```python
from build123d import *

# Parameters (mm, degrees)
SKETCH1_W           = 60
SKETCH1_H           = 12
BOSS_EXTRUDE1_DEPTH = 18.5
SKETCH2_W           = 65
SKETCH2_H           = 6.6
CUT_EXTRUDE1_DEPTH  = 15
SKETCH3_R           = 1.6
CUT_EXTRUDE2_DEPTH  = 38.232378382
CUT_EXTRUDE3_DEPTH  = 37.451886097
FILLET1_R           = 0.7
FILLET3_R           = 0.7
FILLET4_R           = 3
SKETCH5_R           = 1.5
CUT_EXTRUDE4_DEPTH  = 35.073450224
FILLET5_R           = 0.5
SKETCH6_W           = 73.746826028
SKETCH6_H           = 28.597179554
CUT_EXTRUDE5_DEPTH  = 2
SKETCH8_R           = 1.5
BOSS_EXTRUDE2_DEPTH = 0.7


with BuildPart() as part:
    # Sketch1 → Boss-Extrude1 (new body)
    with BuildSketch(Plane.XY):
        Rectangle(SKETCH1_W, SKETCH1_H)
    extrude(amount=BOSS_EXTRUDE1_DEPTH)

    # Sketch2 → Cut-Extrude1 (cut)
    with BuildSketch(Plane.XY.offset(18.5)):
        Rectangle(SKETCH2_W, SKETCH2_H)
    extrude(amount=-CUT_EXTRUDE1_DEPTH, mode=Mode.SUBTRACT)

    # Sketch3 → Cut-Extrude2 (cut, through all)
    with BuildSketch(Plane(origin=(0, 6, 0), x_dir=(1, 0, 0), z_dir=(0, 1, 0))):
        with Locations(Location((25, -15.5, 0), (0, 0, 180))):
            Circle(SKETCH3_R)
        with Locations(Location((-25, -15.5, 0), (0, 0, 180))):
            Circle(SKETCH3_R)
    extrude(amount=-CUT_EXTRUDE2_DEPTH, mode=Mode.SUBTRACT)

    # Sketch4 → Cut-Extrude3 (cut, symmetric)
    with BuildSketch(Plane(origin=(0, -3.3, 0), x_dir=(1, 0, 0), z_dir=(0, 1, 0))):
        Polygon((-30, -3.5), (-28, -18.5), (-30, -18.5), align=None)
    cut_extrude3 = extrude(amount=CUT_EXTRUDE3_DEPTH, both=True, mode=Mode.SUBTRACT)

    # Mirror1: Cut-Extrude3 across plane
    add(cut_extrude3.mirror(Plane(origin=(0, 0, 0), x_dir=(0, 0, 1), z_dir=(1, 0, 0))), mode=Mode.SUBTRACT)

    # Fillet1
    fillet1_edges = [part.edges().sort_by_distance(p)[0] for p in [
        (0, 3.3, 3.5),
        (0, -3.3, 3.5),
    ]]
    fillet(fillet1_edges, radius=FILLET1_R)

    # Fillet3
    fillet3_edges = [part.edges().sort_by_distance(p)[0] for p in [
        (0, -3.3, 18.5),
        (0, -6, 18.5),
        (-28, 4.65, 18.5),
        (-28, -4.65, 18.5),
        (0, 3.3, 18.5),
        (0, 6, 18.5),
        (28, 4.65, 18.5),
        (28, -4.65, 18.5),
    ]]
    fillet(fillet3_edges, radius=FILLET3_R)

    # Fillet4
    # the kernel refuses this fillet: 3 mm, written as the material it takes off along each edge
    with BuildSketch(Plane(origin=(30, -6, -18), x_dir=(-1, 0, 0), z_dir=(0, 0, 1)), Plane(origin=(-30, -6, -18), x_dir=(0, 1, 0), z_dir=(0, 0, 1))) as fillet4_piece_1:
        with BuildLine():
            CenterArc((FILLET4_R, -FILLET4_R), FILLET4_R, 90, 90)
            Line((0, -FILLET4_R), (-FILLET4_R * 0.02, -FILLET4_R))
            Line((-FILLET4_R * 0.02, -FILLET4_R), (-FILLET4_R * 0.02, FILLET4_R * 0.02))
            Line((-FILLET4_R * 0.02, FILLET4_R * 0.02), (FILLET4_R, FILLET4_R * 0.02))
            Line((FILLET4_R, FILLET4_R * 0.02), (FILLET4_R, 0))
        make_face()
    extrude(amount=39.5, mode=Mode.SUBTRACT)
    with BuildSketch(Plane(origin=(30, 6, -18), x_dir=(-1, 0, 0), z_dir=(0, 0, 1)), Plane(origin=(-30, 6, -18), x_dir=(0, -1, 0), z_dir=(0, 0, 1))) as fillet4_piece_2:
        with BuildLine():
            CenterArc((FILLET4_R, FILLET4_R), FILLET4_R, 180, 90)
            Line((0, FILLET4_R), (-FILLET4_R * 0.02, FILLET4_R))
            Line((-FILLET4_R * 0.02, FILLET4_R), (-FILLET4_R * 0.02, -FILLET4_R * 0.02))
            Line((-FILLET4_R * 0.02, -FILLET4_R * 0.02), (FILLET4_R, -FILLET4_R * 0.02))
            Line((FILLET4_R, -FILLET4_R * 0.02), (FILLET4_R, 0))
        make_face()
    extrude(amount=39.5, mode=Mode.SUBTRACT)

    # Sketch5 → Cut-Extrude4 (cut, through all)
    with BuildSketch(Plane.XY.offset(3.5)):
        with Locations((-25, 0)):
            Circle(SKETCH5_R)
        with Locations((25, 0)):
            Circle(SKETCH5_R)
    extrude(amount=-CUT_EXTRUDE4_DEPTH, mode=Mode.SUBTRACT)

    # Fillet5
    fillet5_edges = [part.edges().sort_by_distance(p)[0] for p in [
        (-26.5, 0, 3.5),
        (23.5, 0, 3.5),
    ]]
    fillet(fillet5_edges, radius=FILLET5_R)

    # Sketch6 → Cut-Extrude5 (cut)
    with BuildSketch(Plane.XY):
        Rectangle(SKETCH6_W, SKETCH6_H)
    extrude(amount=CUT_EXTRUDE5_DEPTH, mode=Mode.SUBTRACT)

    # Sketch8 → Boss-Extrude2 (add)
    with BuildSketch(Plane(origin=(0, 0, 2), x_dir=(-1, 0, 0), z_dir=(0, 0, -1))):
        with BuildLine():
            Line((28, -8), (-28, -8))
            ThreePointArc((-28, -8), (-31.535533906, -6.535533906), (-33, -3))
            Line((-33, -3), (-33, 3))
            ThreePointArc((-33, 3), (-31.535533906, 6.535533906), (-28, 8))
            Line((-28, 8), (28, 8))
            ThreePointArc((28, 8), (31.535533906, 6.535533906), (33, 3))
            Line((33, 3), (33, -3))
            ThreePointArc((33, -3), (31.535533906, -6.535533906), (28, -8))
        make_face()
        with Locations(Location((-25, 0, 0), (0, 0, 180))):
            Circle(SKETCH8_R, mode=Mode.SUBTRACT)
        with Locations(Location((25, 0, 0), (0, 0, 180))):
            Circle(SKETCH8_R, mode=Mode.SUBTRACT)
    extrude(amount=BOSS_EXTRUDE2_DEPTH)


solid = part.part
```
Design review of the part built by this model. Coordinates are the model's own, in mm. A direction names the side the tool comes from. Give positions to 0.01 mm unless a question says otherwise; leave off trailing zeros. Write each loop counter-clockwise with the first axis right and the second up, starting at its lowest first coordinate (ties: lowest second). Pieces come first, ordered by that corner, then holes. Notation, with made-up numbers: (-37, 73) - (7, 73) arc R36 ccw to (7, 111) - close; hole circle Ø6 at (13.25, 40.5). An arc over 180 degrees is marked (long way). Return JSON: item names as keys, results as strings. Group by question number.
(1) We need section D-D, the plane x = 14. Give the boundary of the cut face in (y, z), then the cut area to 3 significant figures.
(2) Mouldability with a two-part tool opening along Y and no side actions: class faces 6 (the flat face through (30, 0, 3)), 7 (the flat face through (0, 3.3, 11)), 8 (the cylindrical face through (28.298, 5.705, 8.199)) as +Y half, -Y half, draft (parallel to the pull), parting line (faces both ways), or undercut.
(3) To check wall thickness, follow probe 1 along Y at (x, z) = (-20, 9); probe 2 along Z at (x, y) = (25, 4.75); probe 3 along Y at (x, z) = (-25, 1.9). State the ranges of each line that lie inside material, in increasing order.
(4) We need section B-B, the plane y = 0. Give the boundary of the cut face in (x, z).
(5) We need section A-A, the plane x = 25. Give the number of separate pieces and of enclosed holes in the cut face, then the cut area to 3 significant figures.
(6) Insertion check: pin 1 (1 mm diameter, centred on y = -4, z = 8.5, fed in from -X); pin 2 (1 mm diameter, centred on x = -16.5, z = 5.5, fed in from -Y); pin 3 (5 mm diameter, centred on y = -6.5, z = 11.5, fed in from -X). Each pin has a flat end and moves straight along its axis. Give the tip position at first contact, or say it passes through.
(7) Machinability: for faces 1 (the flat face through (28.84, 4.22, 12.19)), 2 (the cylindrical face through (-28.24, 5.73, 8.2)), 3 (the flat face through (0, 6, 10)), 4 (the flat face through (0, -3.3, 11)), 5 (the cylindrical face through (-28.298, -5.705, 8.199)), which of the approach directions +Z, -Z, +X, -X, +Y, -Y give a long, thin tool a straight path to every point of the face, cutting with its end or side? Answer none if there is none.
(8) We need section C-C, the plane z = 8.25. Give the boundary of the cut face in (x, y).
Reported:
{
 "1": {"outline": "(-8, 1.3) - (8, 1.3) - (8, 2) - (6, 2) - (6, 17.8) arc R0.7 ccw to (5.3, 18.5) - (4, 18.5) arc R0.7 ccw to (3.3, 17.8) - (3.3, 4.2) arc R0.7 cw to (2.6, 3.5) - (-2.6, 3.5) arc R0.7 cw to (-3.3, 4.2) - (-3.3, 17.8) arc R0.7 ccw to (-4, 18.5) - (-5.3, 18.5) arc R0.7 ccw to (-6, 17.8) - (-6, 2) - (-8, 2) - close", "area": "110 mm2"},
 "2": {"face 6": "draft", "face 7": "undercut", "face 8": "+Y half"},
 "3": {"probe 1": "y = -6 to -3.3, 3.3 to 6", "probe 2": "z = 1.3 to 13.9, 17.1 to 18.5", "probe 3": "y = -8 to -1.5, 1.5 to 8"},
 "4": {"outline": "(-33, 1.3) - (-26.5, 1.3) - (-26.5, 3) arc R0.5 ccw to (-27, 3.5) - (-30, 3.5) - (-30, 2) - (-33, 2) - close; (-23.5, 1.3) - (23.5, 1.3) - (23.5, 3) arc R0.5 ccw to (23, 3.5) - (-23, 3.5) arc R0.5 ccw to (-23.5, 3) - close; (26.5, 1.3) - (33, 1.3) - (33, 2) - (30, 2) - (30, 3.5) - (27, 3.5) arc R0.5 ccw to (26.5, 3) - close"},
 "5": {"separate pieces": "4", "enclosed holes": "0", "area": "86.0 mm2"},
 "6": {"pin 1": "stops at x = -29.4", "pin 2": "stops at y = -6", "pin 3": "stops at x = -29.2"},
 "7": {"face 1": "+Z, +X, +Y, -Y", "face 2": "+Z, -X, +Y", "face 3": "+Z, +X, -X, +Y", "face 4": "+Z, +X, -X", "face 5": "+Z, -X, -Y"},
 "8": {"outline": "(-29.37, -4.84) arc R3 ccw to (-27, -6) - (27, -6) arc R3 ccw to (29.37, -4.84) - (29.37, -3.3) - (-29.37, -3.3) - close; (-29.37, 3.3) - (29.37, 3.3) - (29.37, 4.84) arc R3 ccw to (27, 6) - (-27, 6) arc R3 ccw to (-29.37, 4.84) - close"}
}
